Autodesk Inventor part; units mm, degrees
ref_plane "YZ Plane" through (0, 0, 0) normal (1, 0, 0) x (0, 1, 0)
ref_plane "XZ Plane" through (0, 0, 0) normal (0, 1, 0) x (-1, 0, 0)
ref_plane "XY Plane" through (0, 0, 0) normal (0, 0, 1) x (1, 0, 0)
sketch "Sketch1" plane through (0, 0, 0) normal (0, 0, 1) x (1, 0, 0)
  line L0 (0, 0) -> (130.3782, 0)
  line L1 (130.3782, 0) -> (130.3782, 43.815)
  line L2 (130.3782, 43.815) -> (0, 43.815)
  line L3 (0, 43.815) -> (0, 0)
  dimension "d0" = 130.3782
  dimension "d1" = 43.815
extrude "Extrusion1" add sketch "Sketch1" along normal blind 1.651
sketch "Sketch2" plane through (0, 0, 0) normal (0, 0, -1) x (-1, 0, 0)
  circle A0 centre (-110.162, 38.5548) radius 3.25
  circle A1 centre (-68.9426, 35.1048) radius 1.75
  circle A2 centre (-57.5127, 35.1048) radius 1.75
  circle A3 centre (-110.162, 38.5548) radius 3.758
  circle A4 centre (-68.9426, 35.1048) radius 3.8074
  circle A5 centre (-57.5127, 35.1048) radius 3.8074
  point P0 (0, 0)
  dimension "d4" = 0.508
  dimension "d5" = 3.5
  dimension "d6" = 2.0574
  dimension "d7" = 2.0574
extrude "Extrusion2" cut sketch "Sketch2" against normal blind 1.651 contours A0 | A1 | A2 | A3 | A4 | A5
fillet "Fillet1" radius 0.7937 3 edges at (113.92, 38.5548, 0) (72.75, 35.1048, 0) (61.3201, 35.1048, 0)
properties part number "back_plate"
Source: CAD feature listing. Evaluate the final solid. Frame: model axes, mm. Give positions to 0.01 mm unless a question says otherwise; leave off trailing zeros. Order: outer loops, then holes, each group sorted by start corner. A loop starts at its lowest first (then second) coordinate and runs counter-clockwise, first axis right, second up.
(1) Pull-direction query (Y, two-part tool) for faces 1 (the face through (112.932, 41.095, 1.216)), 2 (the face through (64, 22, 1.651)); classes: +Y half, -Y half, draft (parallel to the pull), parting line (faces both ways), or undercut.
(2) Material intervals for line 1 along X through (y, z) = (38, 0.95); line 2 along Y through (x, z) = (70, 1) (3 decimals); line 3 along Y through (x, z) = (55, 0.9) (3 decimals), sorted ascending.
(3) Section query A-A (z = 0.4). Return the cut outline in (x, y) (3 decimals).
(4) Contact query for a flat-ended pin moving along its axis: P1, Ø6, axis at x = 68.94, y = 35.1, coming from the +Z side. Output: stop coordinate, or through.
(5) Section query B-B (y = 37). State how many separate pieces and enclosed holes the cut face has, plus the area to 3 significant figures.
Outcome:
1. face 1: undercut
1. face 2: draft
2. line 1: x = 0 to 55.04, 59.99 to 66.47, 71.42 to 106.45, 113.88 to 130.38
2. line 2: y = 0 to 31.447, 38.762 to 43.815
2. line 3: y = 0 to 32.244, 37.965 to 43.815
3. outline: (0, 0) - (130.378, 0) - (130.378, 43.815) - (0, 43.815) - close; hole circle Ø7.824 at (57.513, 35.105); hole circle Ø7.824 at (68.943, 35.105); hole circle Ø7.725 at (110.162, 38.555)
4. P1: passes through
5. separate pieces: 4
5. enclosed holes: 0
5. area: 181 mm2
